Input: part model. Units: mm. Frame: model coordinates. A direction names the side the tool comes from. Coordinates: 2 decimals unless noted, no trailing zeros. Write each loop counter-clockwise with the first axis right and the second up, starting at its lowest first coordinate (ties: lowest second). Pieces come first, ordered by that corner, then holes. Notation, with made-up numbers: (-19, -11.5) -> (20, -11.5) arc R25 cw to (20, 5.5) -> close; hole circle Ø2 at (24, 73). An arc over 180 degrees is marked (long way). Use one line per item in the form item = value. Start each with the question number.
(1) Cut plane C-C on x = -11.5. Return the cut outline in (y, z), plus the area to 3 significant figures.
(2) Cut plane A-A on x = 0. Return the cut outline in (y, z).
(3) Ray query, line 1 along Y through (x, z) = (23.5, 3.5); line 2 along X through (y, z) = (-1.25, 8.5); line 3 along Z through (x, y) = (16, -6.5). Return the intervals inside material, ascending.
(4) Cut plane D-D on x = -26. Return the cut outline in (y, z).
(5) Set-up query: faces 5 (the face through (32, -9, 1)), 6 (the face through (-0.033, 7.242, 4.93)), 7 (the face through (25, -5, 3)), 8 (the face through (-26, -5, 3)). Return all of +Z, -Z, +X, -X, +Y, -Y with unobstructed straight access to the full face (end or side cutting, diameter ignored); none if empty.
(6) Pull-direction query (Y, two-part tool) for faces 1 (the face through (7.171, 1.314, 4.93)), 2 (the face through (16.2, -6.7, 7.2)), 3 (the face through (0, -9, 3)), 4 (the face through (27.743, -8.549, 3.044)); classes: released by +Y, released by -Y, zero draft, split by the parting line, or undercut.
(7) Cut plane B-B on y = 3.5. Return the cut outline in (x, z), plus the area to 3 significant figures.
(8) First-contact query: pin 1 (2 mm diameter, centred on x = -15, z = 3.5, fed in from +Y); pin 2 (3 mm diameter, centred on x = -10, z = 4, fed in from +Y); pin 3 (3.5 mm diameter, centred on x = 24.5, y = -9, fed in from +Z). Flat tips, straight axial feed; report the tip coordinate or a pass-through.
```python
from build123d import *

# Parameters (mm, degrees)
BOSS_EXTRU_4_DEPTH      = 10
TROU_TARAUD_M43_REACH   = 29.992
TROU_TARAUD_M43_BORE_R  = 1.65
BOSS_EXTRU_5_DEPTH      = 6
BOSS_EXTRU_8_DEPTH      = 7
CONG_1_R                = 0.5
ENL_V_MAT_EXTRU_1_DEPTH = 46.732281958


with BuildPart() as part:
    # Esquisse5 → Boss.-Extru.4 (new body)
    with BuildSketch(Plane.XY):
        with BuildLine():
            Line((-14.485281374, -1.757359313), (-4.242640687, 8.485281374))
            ThreePointArc((-4.242640687, 8.485281374), (0, 10.242640687), (4.242640687, 8.485281374))
            Line((4.242640687, 8.485281374), (14.485281374, -1.757359313))
            ThreePointArc((14.485281374, -1.757359313), (15.785917882, -8.296100594), (10.242640687, -12))
            Line((10.242640687, -12), (-10.242640687, -12))
            ThreePointArc((-10.242640687, -12), (-15.785917882, -8.296100594), (-14.485281374, -1.757359313))
        make_face()
        with BuildLine():
            Line((10.242640687, -9), (-10.242640687, -9))
            ThreePointArc((-10.242640687, -9), (-13.014279285, -7.148050297), (-12.363961031, -3.878679656))
            Line((-12.363961031, -3.878679656), (-2.121320344, 6.363961031))
            ThreePointArc((-2.121320344, 6.363961031), (0, 7.242640687), (2.121320344, 6.363961031))
            Line((2.121320344, 6.363961031), (12.363961031, -3.878679656))
            ThreePointArc((12.363961031, -3.878679656), (13.014279285, -7.148050297), (10.242640687, -9))
        make_face(mode=Mode.SUBTRACT)
    extrude(amount=BOSS_EXTRU_4_DEPTH)

    # Trou taraudé M43 bore (on position points) → Trou taraudé M43 (cut, up to next)
    with BuildSketch(Plane(origin=(0, -12, 5), x_dir=(0, 0, -1), z_dir=(0, -1, 0)), mode=Mode.PRIVATE) as trou_taraud_m43_sk1:
        Circle(TROU_TARAUD_M43_BORE_R)
    trou_taraud_m43_tool1 = extrude(trou_taraud_m43_sk1.sketch, amount=-TROU_TARAUD_M43_REACH, mode=Mode.PRIVATE) & part.part
    add(trou_taraud_m43_tool1.solids().sort_by_distance((0, -12, 5))[0], mode=Mode.SUBTRACT)

    # Esquisse13 → Boss.-Extru.5 (add)
    with BuildSketch(Plane.XY):
        with BuildLine():
            Line((-10.242640687, -12), (-35.242640687, -12))
            Line((-35.242640687, -12), (-35.242640687, -5))
            Line((-35.242640687, -5), (-16.15872047, -5))
            ThreePointArc((-16.15872047, -5), (-14.825216382, -9.872983346), (-10.242640687, -12))
        make_face()
        with BuildLine():
            Line((10.242640687, -12), (30.242640687, -12))
            Line((30.242640687, -12), (30.242640687, -5))
            Line((30.242640687, -5), (16.15872047, -5))
            ThreePointArc((16.15872047, -5), (14.825216382, -9.872983346), (10.242640687, -12))
        make_face()
    extrude(amount=BOSS_EXTRU_5_DEPTH)

    # Esquisse18 → Boss.-Extru.8 (add)
    with BuildSketch(Plane(origin=(0, -12, 0), x_dir=(-1, 0, 0), z_dir=(0, -1, 0))):
        with BuildLine():
            Line((-30.242640687, 0), (-34.439865049, 0))
            ThreePointArc((-34.439865049, 0), (-36.820225395, 0.452013312), (-38.923796238, -0.750243366))
            Line((-38.923796238, -0.750243366), (-38.157751795, -1.393030976))
            ThreePointArc((-38.157751795, -1.393030976), (-33.742640687, -3), (-38.157751795, -4.606969024))
            Line((-38.157751795, -4.606969024), (-38.923796238, -5.249756634))
            ThreePointArc((-38.923796238, -5.249756634), (-36.820225395, -6.452013312), (-34.439865049, -6))
            Line((-34.439865049, -6), (-30.242640687, -6))
            Line((-30.242640687, -6), (-30.242640687, 0))
        make_face()
    extrude(amount=-BOSS_EXTRU_8_DEPTH)

    # Congé1
    cong_1_edges = [part.edges().sort_by_distance(p)[0] for p in [
        (38.157751795, -8.5, 1.393030976),
        (38.923796238, -8.5, 0.750243366),
        (38.923796238, -8.5, 5.249756634),
        (38.157751795, -8.5, 4.606969024),
    ]]
    fillet(cong_1_edges, radius=CONG_1_R - 0.0001)  # a hair under: the kernel refuses the full size

    # Esquisse19 → Enlèv. mat.-Extru.1 (cut, through all)
    with BuildSketch(Plane.XZ.offset(12)):
        with BuildLine():
            Line((29.742640687, 1), (34.742640687, 1))
            ThreePointArc((34.742640687, 1), (33.742640687, 3), (34.742640687, 5))
            Line((34.742640687, 5), (29.742640687, 5))
            ThreePointArc((29.742640687, 5), (27.742640687, 3), (29.742640687, 1))
        make_face()
    extrude(amount=-ENL_V_MAT_EXTRU_1_DEPTH, mode=Mode.SUBTRACT)


solid = part.part
```
Values:
q1.outline = (-12, 0) -> (-8.72, 0) -> (-8.72, 10) -> (-11.87, 10) -> (-11.87, 6) -> (-12, 6) -> close; (-3.01, 0) -> (1.23, 0) -> (1.23, 10) -> (-3.01, 10) -> close
q1.area = 74.7 mm2
q2.outline = (-12, 0) -> (-9, 0) -> (-9, 3.35) -> (-12, 3.35) -> close; (-12, 6.65) -> (-9, 6.65) -> (-9, 10) -> (-12, 10) -> close; (7.24, 0) -> (10.24, 0) -> (10.24, 10) -> (7.24, 10) -> close
q3.line_1 = -12 to -5
q3.line_2 = -13.98 to -9.74, 9.74 to 13.98
q3.line_3 = 0 to 10
q4.outline = (-12, 0) -> (-5, 0) -> (-5, 6) -> (-12, 6) -> close
q5.face_5 = +Y, -Y
q5.face_6 = +Z, -Z
q5.face_7 = +Z, -Z, +X, +Y
q5.face_8 = +Z, -Z, -X, +Y
q6.face_1 = undercut
q6.face_2 = split by the parting line
q6.face_3 = undercut
q6.face_4 = zero draft
q7.outline = (-9.23, 0) -> (-4.99, 0) -> (-4.99, 10) -> (-9.23, 10) -> close; (4.99, 0) -> (9.23, 0) -> (9.23, 10) -> (4.99, 10) -> close
q7.area = 84.9 mm2
q8.pin_1 = -1.27
q8.pin_2 = 4.23
q8.pin_3 = 6
